Input: part model. Units: mm. Frame: model coordinates. Coordinates: 2 decimals unless noted, no trailing zeros. Write each loop counter-clockwise with the first axis right and the second up, starting at its lowest first coordinate (ties: lowest second). Pieces come first, ordered by that corner, then holes.
1) Section query C-C (y = -4.25). Output: boundary loops of the cut face in (x, z), then the cut area to 3 significant figures.
2) Section query A-A (x = -98). Output: boundary loops of the cut face in (y, z), then the cut area to 3 significant figures.
3) Pin query (flat end, axial travel): pin 1 Ø1 at (y, z) = (-19.5, 3) entering from -X; pin 2 Ø8 at (y, z) = (-8.5, -4.5) entering from +X; pin 3 Ø8 at (y, z) = (-13, -5.5) entering from -X. Return the tip coordinate at first contact, or that it passes through.
4) Line query: L1, parallel to Z at x = -161, y = -8; L2, parallel to Z at x = -99.5, y = -18; L3, parallel to X at y = -12.5, z = -7. Output: solid intervals per line, ascending.
5) Draft query along Z for faces 1 (the cylindrical face through (-158.14, -10.85, 0.9)), 2 (the cylindrical face through (-101, -11, 0)), 3 (the cylindrical face through (8, -11, 0)), 4 (the flat face through (-79, -11, 8)). Return one class per face: pulls with the +Z half, pulls with the -Z half, needs draft (parallel to the pull), parting line crosses it, or undercut.
6) Section query B-B (z = 0). Output: boundary loops of the cut face in (x, y).
from build123d import *

# Parameters (mm, degrees)
F0_W     = 8
F0_H     = 16
F0_W_2   = 24
F0_R     = 3
F0_W_3   = 35
F1_DEPTH = 6
F2_DEPTH = 22


with BuildPart() as f1:
    # F0 (on Front) → F1 (new body)
    with BuildSketch(Plane.XZ):
        with BuildLine():
            ThreePointArc((0, -8), (5.6568542495, -5.6568542495), (8, 0))
            ThreePointArc((8, 0), (5.6568542495, 5.6568542495), (0, 8))
            Line((0, 8), (0, -8))
        make_face()
        with BuildLine():
            Line((0, -8), (0, 8))
            ThreePointArc((0, 8), (-8, 0), (0, -8))
        make_face()
        with BuildLine():
            ThreePointArc((0, -8), (-8, 0), (0, 8))
            Line((0, 8), (-72, 8))
            Line((-72, 8), (-72, -8))
            Line((-72, -8), (0, -8))
        make_face()
        with Locations((-76, 0)):
            Rectangle(F0_W, F0_H)
        with Locations((-92, 0)):
            Rectangle(F0_W_2, F0_H)
        with Locations((-98, 0)):
            Circle(F0_R, mode=Mode.SUBTRACT)
        with Locations((-108, 0)):
            Rectangle(F0_W, F0_H)
        with Locations((-129.5, 0)):
            Rectangle(F0_W_3, F0_H)
        with Locations((-151, 0)):
            Rectangle(F0_W, F0_H)
        with BuildLine():
            Line((-155, -8), (-155, 8))
            Line((-155, 8), (-161, 8))
            ThreePointArc((-161, 8), (-169, 0), (-161, -8))
            Line((-161, -8), (-155, -8))
        make_face()
        with Locations((-161, 0)):
            Circle(F0_R, mode=Mode.SUBTRACT)
    extrude(amount=F1_DEPTH)

    # F0 (on Front) → F2 (join)
    with BuildSketch(Plane.XZ):
        with BuildLine():
            ThreePointArc((0, -8), (5.6568542495, -5.6568542495), (8, 0))
            ThreePointArc((8, 0), (5.6568542495, 5.6568542495), (0, 8))
            Line((0, 8), (0, -8))
        make_face()
        with BuildLine():
            Line((0, -8), (0, 8))
            ThreePointArc((0, 8), (-8, 0), (0, -8))
        make_face()
        with BuildLine():
            ThreePointArc((0, -8), (-8, 0), (0, 8))
            Line((0, 8), (-72, 8))
            Line((-72, 8), (-72, -8))
            Line((-72, -8), (0, -8))
        make_face()
        with Locations((-76, 0)):
            Rectangle(F0_W, F0_H)
        with Locations((-92, 0)):
            Rectangle(F0_W_2, F0_H)
        with Locations((-98, 0)):
            Circle(F0_R, mode=Mode.SUBTRACT)
        with Locations((-108, 0)):
            Rectangle(F0_W, F0_H)
        with Locations((-129.5, 0)):
            Rectangle(F0_W_3, F0_H)
        with Locations((-151, 0)):
            Rectangle(F0_W, F0_H)
        with BuildLine():
            Line((-155, -8), (-155, 8))
            Line((-155, 8), (-161, 8))
            ThreePointArc((-161, 8), (-169, 0), (-161, -8))
            Line((-161, -8), (-155, -8))
        make_face()
        with Locations((-161, 0)):
            Circle(F0_R, mode=Mode.SUBTRACT)
    extrude(amount=F2_DEPTH)


solid = f1.part
Answer:
1. outline: (-161, -8) - (0, -8) arc R8 ccw to (0, 8) - (-161, 8) arc R8 ccw to start; hole circle Ø6 at (-161, 0); hole circle Ø6 at (-98, 0)
1. area: 2,720 mm2
2. outline: (-22, -8) - (0, -8) - (0, -3) - (-22, -3) - close; (-22, 3) - (0, 3) - (0, 8) - (-22, 8) - close
2. area: 220 mm2
3. pin 1: stops at x = -168.6
3. pin 2: stops at x = 7.98
3. pin 3: stops at x = -168.86
4. L1: z = -8 to -3, 3 to 8
4. L2: z = -8 to -2.6, 2.6 to 8
4. L3: x = -164.87 to 3.87
5. face 1: undercut
5. face 2: undercut
5. face 3: parting line crosses it
5. face 4: pulls with the +Z half
6. outline: (-169, -22) - (-164, -22) - (-164, 0) - (-169, 0) - close; (-158, -22) - (-101, -22) - (-101, 0) - (-158, 0) - close; (-95, -22) - (8, -22) - (8, 0) - (-95, 0) - close
